Geometry check sheet. Reference: the model listing, model coordinates, mm. A direction names the side the tool comes from. Give positions to 0.01 mm unless a question says otherwise; leave off trailing zeros. Order: outer loops, then holes, each group sorted by start corner. A loop starts at its lowest first (then second) coordinate and runs counter-clockwise, first axis right, second up. Notation, with made-up numbers: M -39.5,85.25 L -9.5,85.25 A25 ccw -9.5,119.25 Z; hole C 20,82 d7. An arc over 180 degrees is marked long. Answer as CSV lines item,"result". Start each with the question number.
Q1. Mould release check, pull along Z, two halves, no side actions. Record for faces 1 (the flat face through (1.5, 5, 26)), 2 (the cylindrical face through (0.74, 3.278, -123.837)), 3 (the cylindrical face through (0.74, 6.07, -33.08)): +Z half, -Z half, draft (parallel to the pull), parting line (faces both ways), or undercut.
Q2. Section check B-B, the plane z = -21. Record the boundary of the cut face in (x, y).
Q3. Section check C-C, the plane y = -18. Record the boundary of the cut face in (x, z).
Q4. Thickness scan on line 1 (Z direction, x = 0.7, y = 0); line 2 (Z direction, x = 1.35, y = 4.5); line 3 (Z direction, x = 0.9, y = 7). Record the ranges inside material, lowest first.
Q5. Section check A-A, the plane x = 0.85. Count the separate pieces of the cut face and the enclosed holes in it, then the cut area to 3 significant figures.
Q6. Set-up check for faces 4 (the cylindrical face through (0.74, -10.05, -7.85)), 5 (the cylindrical face through (0.74, 20.91, -3.56)), 6 (the cylindrical face through (0.74, 0.483, 110.086)): record each of +Z, -Z, +X, -X, +Y, -Y from which the full face is reachable in a straight line by a thin tool's end or side.
```python
from build123d import *

# Parameters (mm, degrees)
SKETCH_1_R      = 1.5
SKETCH_1_R_2    = 6.45
SKETCH_1_R_3    = 7.95
SKETCH_1_R_4    = 1.925
EXTRUDE_1_DEPTH = 1.5


with BuildPart() as part:
    # 草圖1 → 填料-伸長1 (new body)
    with BuildSketch(Plane(origin=(0, 0, 0), x_dir=(0, 0, -1), z_dir=(1, 0, 0))):
        with BuildLine():
            ThreePointArc((111.555989952, -8.572011863), (6.374730125, -10.137132711), (-98.230068302, -21.244930328))
            ThreePointArc((-98.230068302, -21.244930328), (-123.67575498, -2.873316644), (-103.541794939, 21.20204032))
            ThreePointArc((-103.541794939, 21.20204032), (5.082777822, 20.871677912), (113.584507189, 15.696576829))
            ThreePointArc((113.584507189, 15.696576829), (123.827345593, 3.028727453), (112.406990492, -8.588743688))
            ThreePointArc((112.406990492, -8.588743688), (111.981133536, -8.59851924), (111.555989952, -8.572011863))
        make_face()
        with Locations((-109.133892688, 10.496301174)):
            Circle(SKETCH_1_R, mode=Mode.SUBTRACT)
        with Locations((-114.613532023, -0.738624405)):
            Circle(SKETCH_1_R, mode=Mode.SUBTRACT)
        with Locations((-107.62362073, -11.101594062)):
            Circle(SKETCH_1_R, mode=Mode.SUBTRACT)
        with Locations((-95.154070101, -10.22963814)):
            Circle(SKETCH_1_R, mode=Mode.SUBTRACT)
        with Locations((-89.674430767, 1.005287439)):
            Circle(SKETCH_1_R, mode=Mode.SUBTRACT)
        with Locations((-96.66434206, 11.368257096)):
            Circle(SKETCH_1_R, mode=Mode.SUBTRACT)
        with Locations((111.605339346, 3.621333032)):
            Circle(SKETCH_1_R_2, mode=Mode.SUBTRACT)
        with Locations((-102.143981395, 0.133331517)):
            Circle(SKETCH_1_R_3, mode=Mode.SUBTRACT)
        with Locations((35.001055541, 5.982881827)):
            Circle(SKETCH_1_R_4, mode=Mode.SUBTRACT)
        with Locations((-44.432813653, 4.686665047)):
            Circle(SKETCH_1_R_4, mode=Mode.SUBTRACT)
    extrude(amount=EXTRUDE_1_DEPTH)


solid = part.part
```
Answer block:
1,face 1,"draft"
1,face 2,"-Z half"
1,face 3,"undercut"
2,outline,"M 0,-9.35 L 1.5,-9.35 L 1.5,20.42 L 0,20.42 Z"
3,outline,"M 0,75.42 L 1.5,75.42 L 1.5,114.37 L 0,114.37 Z"
4,line 1,"z = -123.29 to -116.94, -106.27 to 88.56, 90.79 to 94.2, 110.09 to 113.31, 115.92 to 123.84"
4,line 2,"z = -123.81 to -118, -105.22 to -36.23, -33.77 to 42.52, 46.35 to 95.5, 108.79 to 123.32"
4,line 3,"z = -123.37 to -117.1, -106.11 to -36.64, -33.37 to 98.14, 106.15 to 122.59"
5,separate pieces,"1"
5,enclosed holes,"10"
5,area,"7,410 mm2"
6,face 4,"+X, -X, -Y"
6,face 5,"+X, -X, +Y"
6,face 6,"+X, -X"
